Autodesk Inventor part; units mm, degrees
ref_plane "YZ Plane" through (0, 0, 0) normal (1, 0, 0) x (0, 1, 0)
ref_plane "XZ Plane" through (0, 0, 0) normal (0, 1, 0) x (-1, 0, 0)
ref_plane "XY Plane" through (0, 0, 0) normal (0, 0, 1) x (1, 0, 0)
sketch "Sketch1" plane through (0, 0, 0) normal (1, 0, 0) x (0, 1, 0)
  line L0 (-212.25, 203.2) -> (212.25, 203.2)
  line L1 (212.25, 203.2) -> (212.25, -203.2)
  line L2 (212.25, -203.2) -> (-212.25, -203.2)
  line L3 (-212.25, -203.2) -> (-212.25, 203.2)
  line L4 (-212.25, 203.2) -> (212.25, -203.2) construction
  line L5 (212.25, 203.2) -> (-212.25, -203.2) construction
  point P0 (0, 0)
  dimension "d0" = 406.4
  dimension "d1" = 424.5
extrude "Extrusion1" add sketch "Sketch1" along normal mid plane 12.7
sketch "Sketch2" plane through (6.35, 0, 0) normal (1, 0, 0) x (0, 0, -1)
  circle A0 centre (-63.5, -161.45) radius 5
  line L0 (203.2, -212.25) -> (203.2, 212.25)
  line L1 (203.2, 212.25) -> (-203.2, 212.25)
  line L2 (-203.2, 212.25) -> (-203.2, -212.25)
  line L3 (-203.2, -212.25) -> (203.2, -212.25)
  circle A1 centre (63.5, -161.45) radius 5
  circle A2 centre (-63.5, -110.65) radius 5
  circle A3 centre (63.5, -110.65) radius 5
  point P0 (0, 0)
  dimension "d6" = 127
  dimension "d9" = 50.8
  dimension "d12" = 10
  dimension "d14" = 63.5
  dimension "d15" = 50.8
extrude "Extrusion2" cut sketch "Sketch2" against normal blind 12.7 contours A0 | A1 | A2 | A3
sketch "Sketch3" plane through (-6.35, -212.25, 203.2) normal (0, 0, 1) x (1, 0, 0)
  line L0 (0, 424.5) -> (12.7, 424.5)
  line L1 (12.7, 0) -> (12.7, 424.5)
  line L2 (0, 424.5) -> (12.7, 424.5)
  line L3 (12.7, 424.5) -> (12.7, 254)
  line L4 (12.7, 254) -> (0, 254)
  line L5 (0, 254) -> (0, 424.5)
  point P0 (6.35, 212.25)
  dimension "d20" = 170.5
extrude "Extrusion3" add sketch "Sketch3" along normal blind 50.8
properties part number "Wood-7"
CAD build for the part. Positions are in the model's coordinates, mm. A direction names the side the tool comes from. Round coordinates to 2 decimals unless told otherwise and drop trailing zeros. Loops run counter-clockwise (first coordinate to the right, second up) from the corner with the lowest first, then second, coordinate; pieces in that order, holes last.
(1) Cut at D-D (y = -46). Give the cut face in (x, z), plus the area to 3 significant figures.
(2) Wall check: line 1 along Y through (x, z) = (2.25, -63.5); line 2 along Z through (x, y) = (5.25, 32); line 3 along Y through (x, z) = (3.5, 208). Give the ranges that are in metal, low to high.
(3) Cut at C-C (x = -4). Give the cut face in (y, z), plus the area to 3 significant figures.
(4) Cut at A-A (z = 63.5). Give the cut face in (x, y).
(5) Which spindle directions (+Z, -Z, +X, -X, +Y, -Y) get a long thin tool onto all of the face, cutting with end or side? Do faces 5 (the flat face through (0, 212.25, 22)), 6 (the flat face through (0, 41.75, 228)). Say none if no direction does.
(6) Drop flat-ended pins along their axis: pin 1 (16 mm diameter, centred on y = -110.65, z = -63.5, fed in from -X); pin 2 (4 mm diameter, centred on x = 2.5, z = 237, fed in from -Y); pin 3 (4 mm diameter, centred on x = -1, y = -46, fed in from +Z). Give the stop position or say it passes through.
(7) Two-plate mould, pull along Y, no slides. Class faces 1 (the cylindrical face through (0.09, -166.33, -62.42)), 2 (the flat face through (0, 128, 254)), 3 (the cylindrical face through (0.09, -166.33, 64.58)), 4 (the flat face through (0, -212.25, -3)): +Y half, -Y half, draft (parallel to the pull), parting line (faces both ways), or undercut.
(8) Cut at B-B (y = -110.65). Give the cut face in (x, z).
Findings below:
1. outline: (-6.35, -203.2) - (6.35, -203.2) - (6.35, 203.2) - (-6.35, 203.2) - close
1. area: 5,160 mm2
2. line 1: y = -212.25 to -166.45, -156.45 to -115.65, -105.65 to 212.25
2. line 2: z = -203.2 to 203.2
2. line 3: y = 41.75 to 212.25
3. outline: (-212.25, -203.2) - (212.25, -203.2) - (212.25, 254) - (41.75, 254) - (41.75, 203.2) - (-212.25, 203.2) - close; hole circle Ø10 at (-161.45, -63.5); hole circle Ø10 at (-161.45, 63.5); hole circle Ø10 at (-110.65, -63.5); hole circle Ø10 at (-110.65, 63.5)
3. area: 181,000 mm2
4. outline: (-6.35, -212.25) - (6.35, -212.25) - (6.35, -166.45) - (-6.35, -166.45) - close; (-6.35, -156.45) - (6.35, -156.45) - (6.35, -115.65) - (-6.35, -115.65) - close; (-6.35, -105.65) - (6.35, -105.65) - (6.35, 212.25) - (-6.35, 212.25) - close
5. face 5: +Z, -Z, +X, -X, +Y
5. face 6: +Z, +X, -X, -Y
6. pin 1: stops at x = -6.35
6. pin 2: stops at y = 41.75
6. pin 3: stops at z = 203.2
7. face 1: undercut
7. face 2: draft
7. face 3: undercut
7. face 4: -Y half
8. outline: (-6.35, -203.2) - (6.35, -203.2) - (6.35, -68.5) - (-6.35, -68.5) - close; (-6.35, -58.5) - (6.35, -58.5) - (6.35, 58.5) - (-6.35, 58.5) - close; (-6.35, 68.5) - (6.35, 68.5) - (6.35, 203.2) - (-6.35, 203.2) - close
